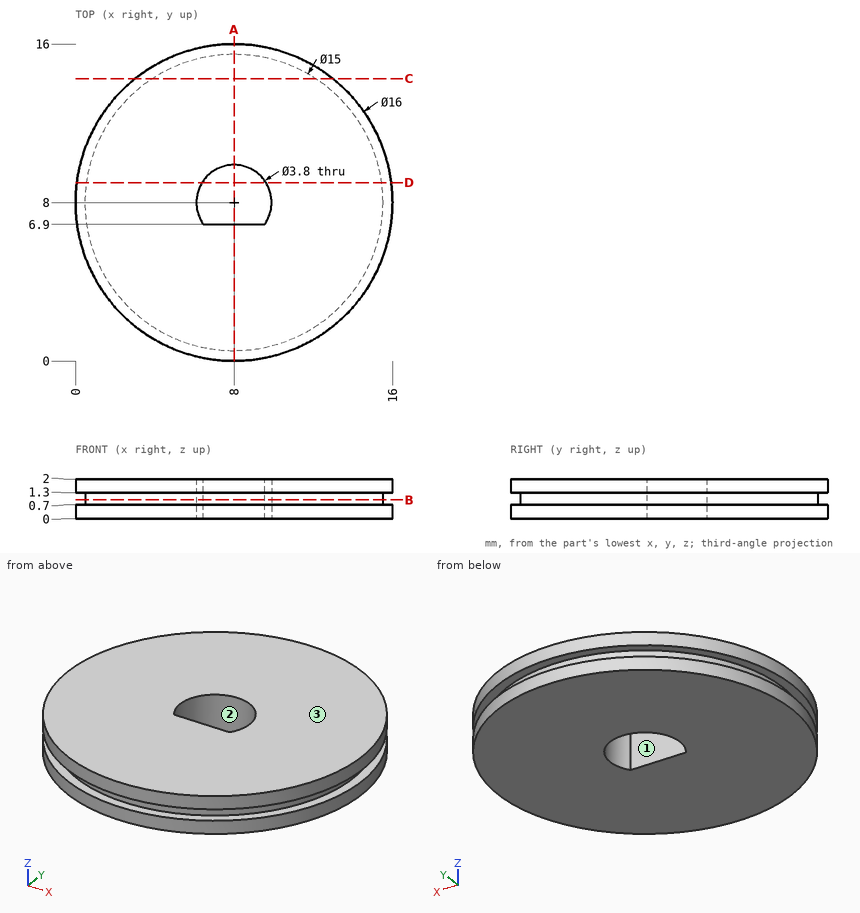
Print and shaded views of the part. All mm, measured from the part's lowest x, y and z. Give positions to 0.01 mm unless a question says otherwise; leave off trailing zeros. Loops run counter-clockwise (first coordinate to the right, second up) from the corner with the lowest first, then second, coordinate; pieces in that order, holes last. Notation, with made-up numbers: (7, 81) -> (53, 81) arc R20 ccw to (53, 86) -> close; hole circle Ø8 at (17, 14.5). An arc over 180 degrees is marked (long way). One line per question, with ' | ' between items. Start each with the question number.
1) Cut at B-B (z = 0.95). Give the cut face in (x, y), plus the area to 3 significant figures.
2) Cut at D-D (y = 9). Give the cut face in (x, z), plus the area to 3 significant figures.
3) Cut at C-C (y = 14.25). Give the cut face in (x, z), plus the area to 3 significant figures.
4) Two-plate mould, pull along Y, no slides. Class the marked faces 1, 2 and 3: released by +Y, released by -Y, zero draft, split by the parting line, or undercut.
5) Cut at A-A (x = 8). Give the cut face in (y, z), plus the area to 3 significant figures.
6) Probe L1, parallel to Z at x = 1.25, y = 12; L2, parallel to Y at x = 8, z = 0.65; L3, parallel to X at y = 8, z = 1.55. List the from-to ranges inside material, lowest first.
Return value:
1) outline: circle Ø15 at (8, 8); hole (6.45, 6.9) -> (9.55, 6.9) arc R1.9 ccw (long way) to start | area: 167 mm^2
2) outline: (0.06, 0) -> (6.38, 0) -> (6.38, 2) -> (0.06, 2) -> (0.06, 1.3) -> (0.57, 1.3) -> (0.57, 0.7) -> (0.06, 0.7) -> close; (9.62, 0) -> (15.94, 0) -> (15.94, 0.7) -> (15.43, 0.7) -> (15.43, 1.3) -> (15.94, 1.3) -> (15.94, 2) -> (9.62, 2) -> close | area: 24.7 mm^2
3) outline: (3.01, 0) -> (12.99, 0) -> (12.99, 0.7) -> (12.15, 0.7) -> (12.15, 1.3) -> (12.99, 1.3) -> (12.99, 2) -> (3.01, 2) -> (3.01, 1.3) -> (3.85, 1.3) -> (3.85, 0.7) -> (3.01, 0.7) -> close | area: 19.0 mm^2
4) face 1: undercut | face 2: undercut | face 3: zero draft
5) outline: (0, 0) -> (6.9, 0) -> (6.9, 2) -> (0, 2) -> (0, 1.3) -> (0.5, 1.3) -> (0.5, 0.7) -> (0, 0.7) -> close; (9.9, 0) -> (16, 0) -> (16, 0.7) -> (15.5, 0.7) -> (15.5, 1.3) -> (16, 1.3) -> (16, 2) -> (9.9, 2) -> close | area: 25.4 mm^2
6) L1: 0 to 0.7, 1.3 to 2 | L2: 0 to 6.9, 9.9 to 16 | L3: 0 to 6.1, 9.9 to 16
